Verification items for the finished model (mm, model axes). Face numbers are marked on the shaded views. A direction names the side the tool comes from. Round coordinates to 2 decimals unless told otherwise and drop trailing zeros. Write each loop counter-clockwise with the first axis right and the second up, starting at its lowest first coordinate (ties: lowest second). Pieces come first, ordered by that corner, then holes. Notation, with made-up numbers: (-31, 66.25) - (-14, 66.25) arc R14 cw to (-14, 70.25) - close; hole circle Ø10 at (83, 45). An arc over 180 degrees is marked (long way). Write each question's results on one line, items separated by ' | '.
```python
from build123d import *

# Parameters (mm, degrees)
SKETCH1_R           = 13
SKETCH1_R_2         = 1.5
BOSS_EXTRUDE1_DEPTH = 2.5
SKETCH2_W           = 69
SKETCH2_H           = 89.5
SKETCH2_W_2         = 65
SKETCH2_H_2         = 85.5
BOSS_EXTRUDE2_DEPTH = 8.85
FILLET1_R           = 5


with BuildPart() as part:
    # Sketch1 → Boss-Extrude1 (new body)
    with BuildSketch(Plane.XY):
        Polygon((0, 0), (10.5, -33), (72.5, -33), (83, 0), (83, 89), (0, 89), align=None)
        with Locations((26, 42.5)):
            Circle(SKETCH1_R, mode=Mode.SUBTRACT)
        with Locations((57, 42.5)):
            Circle(SKETCH1_R, mode=Mode.SUBTRACT)
        with Locations((26, 11.5)):
            Circle(SKETCH1_R, mode=Mode.SUBTRACT)
        with Locations((57, 11.5)):
            Circle(SKETCH1_R, mode=Mode.SUBTRACT)
        with Locations((41.5, 19.99)):
            Circle(SKETCH1_R_2, mode=Mode.SUBTRACT)
    extrude(amount=BOSS_EXTRUDE1_DEPTH)

    # Sketch2 → Boss-Extrude2 (add)
    with BuildSketch(Plane(origin=(0, 0, 0), x_dir=(-1, 0, 0), z_dir=(0, 0, -1))):
        with Locations((-41.5, 36.25)):
            Rectangle(SKETCH2_W, SKETCH2_H)
        with Locations((-41.5, 36.25)):
            Rectangle(SKETCH2_W_2, SKETCH2_H_2, mode=Mode.SUBTRACT)
    extrude(amount=BOSS_EXTRUDE2_DEPTH)

    # Fillet1
    fillet1_edges = [part.edges().sort_by_distance(p)[0] for p in [
        (0, 89, 1.25),
        (83, 89, 1.25),
        (83, 0, 1.25),
        (72.5, -33, 1.25),
        (10.5, -33, 1.25),
        (0, 0, 1.25),
        (74, -6.5, -4.425),
        (74, 79, -4.425),
        (9, 79, -4.425),
        (7, -8.5, -4.425),
        (7, 81, -4.425),
        (76, 81, -4.425),
        (76, -8.5, -4.425),
        (9, -6.5, -4.425),
    ]]
    fillet(fillet1_edges, radius=FILLET1_R)


solid = part.part
```
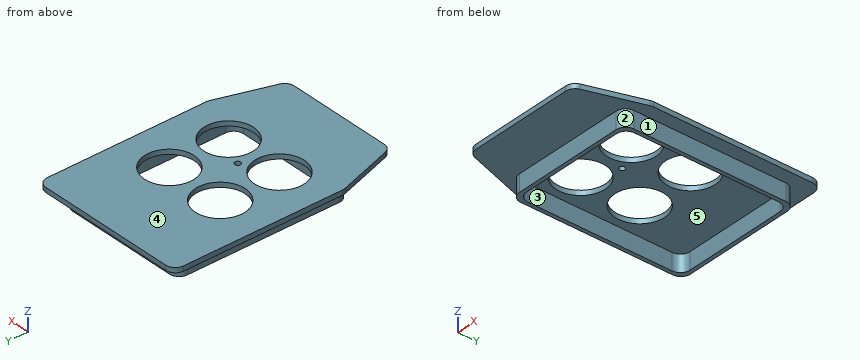
(1) Section check D-D (x = 41.5). Record the cut outline in (y, z).
Answer:
outline: (-33, 0) - (-8.5, 0) - (-8.5, -8.85) - (-6.5, -8.85) - (-6.5, 0) - (18.49, 0) - (18.49, 2.5) - (-33, 2.5) - close; (21.49, 0) - (79, 0) - (79, -8.85) - (81, -8.85) - (81, 0) - (89, 0) - (89, 2.5) - (21.49, 2.5) - close
(2) Section check B-B (y = 42.5). Record the cut outline in (x, z), plus the area to 3 significant figures.
Answer:
outline: (0, 0) - (7, 0) - (7, -8.85) - (9, -8.85) - (9, 0) - (13, 0) - (13, 2.5) - (0, 2.5) - close; (39, 0) - (44, 0) - (44, 2.5) - (39, 2.5) - close; (70, 0) - (74, 0) - (74, -8.85) - (76, -8.85) - (76, 0) - (83, 0) - (83, 2.5) - (70, 2.5) - close | area: 113 mm2
(3) Go/stop test with flat-tipped pins: pin 1 Ø4.5 at (x, z) = (41, -4.5) entering from -Y; pin 2 Ø2.5 at (y, z) = (21.5, -3.5) entering from +X; pin 3 Ø2 at (x, y) = (73, -10) entering from -Z. Record where each tip stops, or that it passes through.
Answer:
pin 1: y = -8.5 | pin 2: x = 76 | pin 3: z = 0
(4) Set-up check for the marked faces 4 and 5: record each of +Z, -Z, +X, -X, +Y, -Y from which the full face is reachable in a straight line by a thin tool's end or side.
Answer:
face 4: +Z, +X, -X, +Y, -Y | face 5: -Z
(5) Section check A-A (x = 57). Record the cut outline in (y, z), plus the area to 3 significant figures.
Answer:
outline: (-33, 0) - (-8.5, 0) - (-8.5, -8.85) - (-6.5, -8.85) - (-6.5, 0) - (-1.5, 0) - (-1.5, 2.5) - (-33, 2.5) - close; (24.5, 0) - (29.5, 0) - (29.5, 2.5) - (24.5, 2.5) - close; (55.5, 0) - (79, 0) - (79, -8.85) - (81, -8.85) - (81, 0) - (89, 0) - (89, 2.5) - (55.5, 2.5) - close | area: 210 mm2
(6) Mould release check, pull along Y, two halves, no side actions. Record for the marked faces 1, 2 and 3: released by +Y, released by -Y, zero draft, split by the parting line, or undercut.
Answer:
face 1: zero draft | face 2: released by -Y | face 3: undercut
(7) Section check C-C (z = -6.5). Record the cut outline in (x, y), plus the area to 3 significant figures.
Answer:
outline: (7, -3.5) arc R5 ccw to (12, -8.5) - (71, -8.5) arc R5 ccw to (76, -3.5) - (76, 76) arc R5 ccw to (71, 81) - (12, 81) arc R5 ccw to (7, 76) - close; hole (9, -1.5) arc R5 ccw to (14, -6.5) - (69, -6.5) arc R5 ccw to (74, -1.5) - (74, 74) arc R5 ccw to (69, 79) - (14, 79) arc R5 ccw to (9, 74) - close | area: 618 mm2
(8) Thickness scan on L1, parallel to Y at x = 57, z = 1.8; L2, parallel to Y at x = 42, z = -7.25; L3, parallel to Y at x = 41.5, z = 1.7. Record the ranges inside material, lowest first.
Answer:
L1: -33 to -1.5, 24.5 to 29.5, 55.5 to 89 | L2: -8.5 to -6.5, 79 to 81 | L3: -33 to 18.49, 21.49 to 89
